Read the model definition and answer for the solid it produces. Units are mm, in the model's axes. Round coordinates to 2 decimals unless told otherwise and drop trailing zeros. Order: outer loops, then holes, each group sorted by start corner. A loop starts at its lowest first (then second) coordinate and runs counter-clockwise, first axis right, second up.
Autodesk Inventor part; units mm, degrees
ref_plane "YZ Plane" through (0, 0, 0) normal (1, 0, 0) x (0, 1, 0)
ref_plane "XZ Plane" through (0, 0, 0) normal (0, 1, 0) x (-1, 0, 0)
ref_plane "XY Plane" through (0, 0, 0) normal (0, 0, 1) x (1, 0, 0)
sketch "Sketch1" plane through (0, 0, 0) normal (0, 1, 0) x (-1, 0, 0)
  line L0 (0, 0) -> (-90, 0)
  line L1 (-162.8128, 0) -> (81.4064, 141)
  line L2 (81.4064, 141) -> (81.4064, -141)
  line L3 (81.4064, -141) -> (-162.8128, 0)
  dimension "d0" = 90
  dimension "d1" = 282
extrude "TriangleFace" add sketch "Sketch1" along normal blind 15
sketch "Sketch2" plane through (0, 15, 0) normal (0, 1, 0) x (1, 0, 0)
  line L0 (-81.4064, 141) -> (-81.4064, -141)
  line L1 (-81.4064, 0) -> (-65.9064, 0)
  line L2 (-65.9064, 0) -> (-65.9064, 20)
  line L3 (-65.9064, 0) -> (-65.9064, -20)
  line L4 (-65.9064, 0) -> (-38.9064, 0)
  line L5 (-38.9064, 0) -> (-38.9064, 20)
  line L6 (-38.9064, 0) -> (-38.9064, -20)
  circle A0 centre (-65.9064, 20) radius 2
  circle A1 centre (-38.9064, 20) radius 2
  circle A2 centre (-65.9064, -20) radius 2
  circle A3 centre (-38.9064, -20) radius 2
  point P0 (0, 0)
  dimension "d4" = 15.5
  dimension "d5" = 20
  dimension "d6" = 20
  dimension "d7" = 27
  dimension "d8" = 20
  dimension "d9" = 20
  dimension "d10" = 4
  dimension "d11" = 4
  dimension "d12" = 4
  dimension "d13" = 4
extrude "SideTwoHoles" cut sketch "Sketch2" against normal blind 15
sketch "Sketch3" plane through (0, 15, 0) normal (0, 1, 0) x (1, 0, 0)
  line L0 (162.8128, 0) -> (-81.4064, 141)
  line L1 (40.7032, 70.5) -> (32.9532, 57.0766)
  line L2 (32.9532, 57.0766) -> (19.4532, 33.6939)
  line L3 (32.9532, 57.0766) -> (15.6327, 67.0766)
  line L4 (32.9532, 57.0766) -> (50.2737, 47.0766)
  line L5 (19.4532, 33.6939) -> (2.1327, 43.6939)
  line L6 (19.4532, 33.6939) -> (36.7737, 23.6939)
  circle A0 centre (15.6327, 67.0766) radius 2
  circle A1 centre (50.2737, 47.0766) radius 2
  circle A2 centre (2.1327, 43.6939) radius 2
  circle A3 centre (36.7737, 23.6939) radius 2
  point P0 (0, 0)
  dimension "d16" = 15.5
  dimension "d17" = 27
  dimension "d18" = 20
  dimension "d19" = 20
  dimension "d20" = 20
  dimension "d21" = 20
  dimension "d22" = 4
  dimension "d23" = 4
  dimension "d24" = 4
  dimension "d25" = 4
extrude "SideOneHoles" cut sketch "Sketch3" against normal blind 15
sketch "Sketch4" plane through (0, 15, 0) normal (0, 1, 0) x (1, 0, 0)
  line L0 (-81.4064, -141) -> (162.8128, 0)
  line L1 (40.7032, -70.5) -> (32.9532, -57.0766)
  line L2 (32.9532, -57.0766) -> (19.4532, -33.6939)
  line L3 (19.4532, -33.6939) -> (36.7737, -23.6939)
  line L4 (19.4532, -33.6939) -> (2.1327, -43.6939)
  line L5 (32.9532, -57.0766) -> (50.2737, -47.0766)
  line L6 (32.9532, -57.0766) -> (15.6327, -67.0766)
  circle A0 centre (36.7737, -23.6939) radius 2
  circle A1 centre (2.1327, -43.6939) radius 2
  circle A2 centre (50.2737, -47.0766) radius 2
  circle A3 centre (15.6327, -67.0766) radius 2
  point P0 (0, 0)
  dimension "d28" = 15.5
  dimension "d29" = 27
  dimension "d30" = 20
  dimension "d31" = 20
  dimension "d32" = 20
  dimension "d33" = 20
  dimension "d34" = 4
  dimension "d35" = 4
  dimension "d36" = 4
  dimension "d37" = 4
extrude "SideThreeHoles" cut sketch "Sketch4" against normal blind 15
sketch "Sketch5" plane through (0, 15, 0) normal (0, 1, 0) x (1, 0, 0)
  line L0 (-81.4064, -141) -> (162.8128, 0)
  line L1 (162.8128, 0) -> (-81.4064, 141)
  line L2 (162.8128, 0) -> (-81.4064, 0)
  line L3 (-81.4064, 141) -> (-81.4064, -141)
  line L4 (17.3205, 0) -> (-8.6603, -15)
  line L5 (-8.6603, -15) -> (-8.6603, 15)
  line L6 (-8.6603, 15) -> (17.3205, 0)
  line L7 (-8.6603, 15) -> (-5.1603, 8.9378)
  line L8 (-8.6603, 15) -> (-1.6603, 15) construction
  circle A0 centre (-5.1603, 8.9378) radius 1.75
  line L9 (-8.6603, -15) -> (-5.1603, -8.9378)
  line L10 (-8.6603, -15) -> (-1.6603, -15) construction
  circle A1 centre (-5.1603, -8.9378) radius 1.75
  line L11 (17.3205, 0) -> (10.3205, 0)
  line L12 (17.3205, 0) -> (24.3205, 0) construction
  circle A2 centre (10.3205, 0) radius 1.75
  point P0 (0, 0)
  point P1 (0, 0)
  dimension "d40" = 30
  dimension "d43" = 7
  dimension "d44" = 60
  dimension "d45" = 3.5
  dimension "d46" = 7
  dimension "d47" = 60
  dimension "d48" = 3.5
  dimension "d49" = 7
  dimension "d50" = 180
  dimension "d51" = 3.5
extrude "CenterHoles" cut sketch "Sketch5" against normal blind 15 contours A1 | A0 | A2 L2 | L2 A2
sketch "Sketch6" plane through (0, 15, 0) normal (0, 1, 0) x (1, 0, 0)
  line L0 (-81.4064, -141) -> (162.8128, 0)
  line L1 (-81.4064, -141) -> (-81.4064, -71)
  line L2 (-81.4064, 141) -> (-81.4064, -141)
  line L3 (-81.4064, -71) -> (-51.4064, -71)
  line L4 (-81.4064, -71) -> (-51.4064, -71) construction
  circle A0 centre (-51.4064, -71) radius 2
  line L5 (162.8128, 0) -> (-81.4064, 141)
  line L6 (-81.4064, 141) -> (-20.7846, 106)
  line L7 (-20.7846, 106) -> (-35.7846, 80.0192)
  line L8 (162.8128, 0) -> (102.191, -35)
  line L9 (102.191, -35) -> (87.191, -9.0192)
  circle A1 centre (-35.7846, 80.0192) radius 2
  circle A2 centre (87.191, -9.0192) radius 2
  point P0 (0, 0)
  dimension "d54" = 70
  dimension "d55" = 30
  dimension "d56" = 0
  dimension "d57" = 4
  dimension "d60" = 70
  dimension "d61" = 30
  dimension "d62" = 70
  dimension "d63" = 30
  dimension "d64" = 4
  dimension "d65" = 4
extrude "Extrusion7" cut sketch "Sketch6" against normal blind 15 contours A2 | A1 | A0
properties part number "TraingleFifteen"
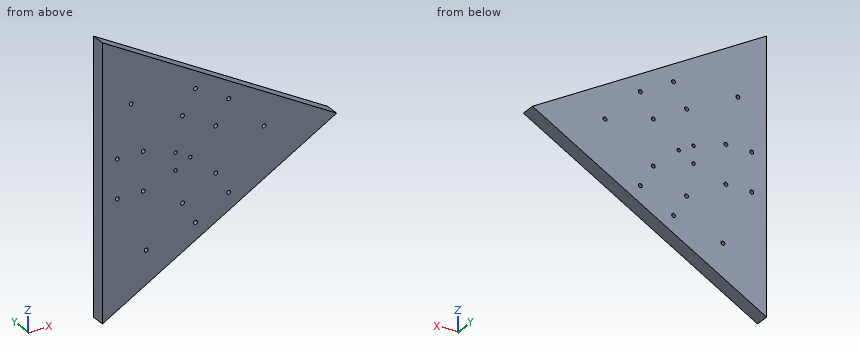
Q1. A cutting plane is placed at C-C, the plane x = 25. Give the vertices of the cut face in (y, z), plus the area to 3 significant figures.
Outcome:
outline: (0, -79.57) - (15, -79.57) - (15, 79.57) - (0, 79.57) - close
area: 2,390 mm2
Q2. Flat-ended cylindrical pins translate along their axes: pin 1 (1.5 mm diameter, centred on x = 77, y = 3, fed in from -Z); pin 2 (2.5 mm diameter, centred on x = 15.63, z = -67.08, fed in from +Y); pin 3 (3 mm diameter, centred on x = 110.5, y = 9, fed in from -Z); pin 4 (5 mm diameter, centred on x = -30, y = 7, fed in from +Z). Find the tip coordinate at first contact, or state that the pin passes through.
Outcome:
pin 1: stops at z = -49.98
pin 2: passes through
pin 3: stops at z = -31.07
pin 4: stops at z = 112.76
Q3. Straight lines are drawn through the part: probe 1 along Z at (x, y) = (16, 11.5); probe 2 along X at (y, z) = (8.25, -44); probe 3 along Z at (x, y) = (-35, 6.25). For each, find the intervals that lie inside material, in ascending order.
Outcome:
probe 1: z = -84.76 to -69.04, -65.11 to 65.11, 69.04 to 84.76
probe 2: x = -81.41 to 0.16, 4.11 to 86.6
probe 3: z = -114.21 to -81.86, -78.18 to 114.21
Q4. A cutting plane is placed at A-A, the plane y = 6.5. Give the number of separate pieces and of enclosed holes in the cut face, plus the area to 3 significant figures.
Outcome:
separate pieces: 1
enclosed holes: 18
area: 34,200 mm2
Q5. A cutting plane is placed at B-B, the plane z = 98.5. Give the vertices of the cut face in (x, y).
Outcome:
outline: (-81.41, 0) - (-7.79, 0) - (-7.79, 15) - (-81.41, 15) - close
